from build123d import *

# Parameters (mm, degrees)
SKETCH1_W                           = 106
SKETCH1_H                           = 106
MAINOUTLINE_DEPTH                   = 1.6
SKETCH4_W                           = 11.7
SKETCH4_H                           = 11.7
RAILCUTOUTS_DEPTH                   = 2.6
FILLETCUTOUTS_START                 = -2.6
SKETCH13_W                          = 5.7
SKETCH13_H                          = 1.9
SKETCH13_W_2                        = 1.8
SKETCH13_H_2                        = 3
FILLETCUTOUTS_DEPTH                 = 3.6
SMOOTHCORNER_DEPTH                  = 10
MIRROR2_COPY_1_SKETCH_W             = 11.7
MIRROR2_COPY_1_SKETCH_H             = 11.7
MIRROR2_COPY_1_DEPTH                = 2.6
MIRROR2_START                       = -2.6
MIRROR2_COPY_2_SKETCH_W             = 5.7
MIRROR2_COPY_2_SKETCH_H             = 1.9
MIRROR2_COPY_2_SKETCH_W_2           = 1.8
MIRROR2_COPY_2_SKETCH_H_2           = 3
MIRROR2_COPY_2_DEPTH                = 3.6
MIRROR2_COPY_3_DEPTH                = 10
MIRROR2_COPY_4_SKETCH_W             = 11.7
MIRROR2_COPY_4_SKETCH_H             = 11.7
MIRROR2_COPY_4_DEPTH                = 2.6
MIRROR2_COPY_5_SKETCH_W             = 5.7
MIRROR2_COPY_5_SKETCH_H             = 1.9
MIRROR2_COPY_5_SKETCH_W_2           = 1.8
MIRROR2_COPY_5_SKETCH_H_2           = 3
MIRROR2_COPY_5_DEPTH                = 3.6
M2_CLEARANCE_HOLE1_D                = 2.1
SKETCH12_R                          = 0.8
INTERBOARDCONNECTORHOLES_DEPTH      = 1
INTERBOARDCONNECTORHOLES_DEPTH_BACK = 2.6
SKETCH16_W                          = 90
SKETCH16_H                          = 6.2
SKETCH16_W_2                        = 5.2
SKETCH16_H_2                        = 90
CUT_EXTRUDE6_DEPTH                  = 0.001
SKETCH21_R                          = 22.5
CUT_EXTRUDE10_DEPTH                 = 2.6
CUT_EXTRUDE10_DEPTH_BACK            = 1
F_2U_TURNSTILE_CUTOUT_REACH         = 3.6
SKETCH24_OUTSIDE_W                  = 137.984
SKETCH24_OUTSIDE_H                  = 137.984
SKETCH24_OUTSIDE_W_2                = 105.6
SKETCH24_OUTSIDE_H_2                = 105.6
CUT_EXTRUDE19_DEPTH                 = 2.6
FILLET7_R                           = 0.5
FILLET8_R                           = 1


with BuildPart() as part:
    # Sketch1 → mainOutline (new body)
    with BuildSketch(Plane.XY):
        Rectangle(SKETCH1_W, SKETCH1_H)
    extrude(amount=MAINOUTLINE_DEPTH)

    # Sketch4 → railCutouts (cut, through all)
    with BuildSketch(Plane(origin=(0, 0, 0), x_dir=(-1, 0, 0), z_dir=(0, 0, -1))):
        with Locations((47.15, 47.15)):
            Rectangle(SKETCH4_W, SKETCH4_H)
    railcutouts = extrude(amount=-RAILCUTOUTS_DEPTH, mode=Mode.SUBTRACT)

    # Sketch13 → filletCutouts (cut)
    with BuildSketch(Plane(origin=(0, 0, 0), x_dir=(-1, 0, 0), z_dir=(0, 0, -1)).offset(FILLETCUTOUTS_START)):
        with Locations((50.15, 40.35)):
            Rectangle(SKETCH13_W, SKETCH13_H)
        with Locations((40.4, 51.5)):
            Rectangle(SKETCH13_W_2, SKETCH13_H_2)
    filletcutouts = extrude(amount=FILLETCUTOUTS_DEPTH, mode=Mode.SUBTRACT)

    # Sketch27 → smoothCorner (cut)
    with BuildSketch(Plane.XY.offset(1.6)):
        with BuildLine():
            Line((-40.928025612, 42.198025612), (-40.928025612, 49.628025612))
            Line((-40.928025612, 49.628025612), (-40.398025612, 49.628025612))
            ThreePointArc((-40.398025612, 49.628025612), (-39.5, 50), (-39.128025612, 50.898025612))
            Line((-39.128025612, 50.898025612), (-39.128025612, 53))
            Line((-39.128025612, 53), (-53, 53))
            Line((-53, 53), (-53, 39.028025612))
            Line((-53, 39.028025612), (-48.198025612, 39.028025612))
            ThreePointArc((-48.198025612, 39.028025612), (-47.3, 39.4), (-46.928025612, 40.298025612))
            Line((-46.928025612, 40.298025612), (-46.928025612, 40.928025612))
            Line((-46.928025612, 40.928025612), (-42.198025612, 40.928025612))
            ThreePointArc((-42.198025612, 40.928025612), (-41.3, 41.3), (-40.928025612, 42.198025612))
        make_face()
    smoothcorner = extrude(amount=-SMOOTHCORNER_DEPTH, mode=Mode.SUBTRACT)

    # Mirror1: railCutouts, filletCutouts, smoothCorner across plane
    add(railcutouts.mirror(Plane(origin=(0, 0, 0), x_dir=(0, 0, 1), z_dir=(1, 0, 0))), mode=Mode.SUBTRACT)
    add(filletcutouts.mirror(Plane(origin=(0, 0, 0), x_dir=(0, 0, 1), z_dir=(1, 0, 0))), mode=Mode.SUBTRACT)
    add(smoothcorner.mirror(Plane(origin=(0, 0, 0), x_dir=(0, 0, 1), z_dir=(1, 0, 0))), mode=Mode.SUBTRACT)

    # Mirror2: smoothCorner across plane
    add(smoothcorner.mirror(Plane.ZX), mode=Mode.SUBTRACT)

    # Mirror2 copy 1 sketch → Mirror2 copy 1 (cut, through all)
    with BuildSketch(Plane(origin=(0, 0, 0), x_dir=(1, 0, 0), z_dir=(0, 0, -1))):
        with Locations((47.15, 47.15)):
            Rectangle(MIRROR2_COPY_1_SKETCH_W, MIRROR2_COPY_1_SKETCH_H)
    extrude(amount=-MIRROR2_COPY_1_DEPTH, mode=Mode.SUBTRACT)

    # Mirror2 copy 2 sketch → Mirror2 copy 2 (cut)
    with BuildSketch(Plane(origin=(0, 0, 0), x_dir=(1, 0, 0), z_dir=(0, 0, -1)).offset(MIRROR2_START)):
        with Locations((50.15, 40.35)):
            Rectangle(MIRROR2_COPY_2_SKETCH_W, MIRROR2_COPY_2_SKETCH_H)
        with Locations((40.4, 51.5)):
            Rectangle(MIRROR2_COPY_2_SKETCH_W_2, MIRROR2_COPY_2_SKETCH_H_2)
    extrude(amount=MIRROR2_COPY_2_DEPTH, mode=Mode.SUBTRACT)

    # Mirror2 copy 3 sketch → Mirror2 copy 3 (cut)
    with BuildSketch(Plane(origin=(0, 0, 1.6), x_dir=(-1, 0, 0), z_dir=(0, 0, 1))):
        with BuildLine():
            Line((-40.928025612, 42.198025612), (-40.928025612, 49.628025612))
            Line((-40.928025612, 49.628025612), (-40.398025612, 49.628025612))
            ThreePointArc((-40.398025612, 49.628025612), (-39.5, 50), (-39.128025612, 50.898025612))
            Line((-39.128025612, 50.898025612), (-39.128025612, 53))
            Line((-39.128025612, 53), (-53, 53))
            Line((-53, 53), (-53, 39.028025612))
            Line((-53, 39.028025612), (-48.198025612, 39.028025612))
            ThreePointArc((-48.198025612, 39.028025612), (-47.3, 39.4), (-46.928025612, 40.298025612))
            Line((-46.928025612, 40.298025612), (-46.928025612, 40.928025612))
            Line((-46.928025612, 40.928025612), (-42.198025612, 40.928025612))
            ThreePointArc((-42.198025612, 40.928025612), (-41.3, 41.3), (-40.928025612, 42.198025612))
        make_face()
    extrude(amount=-MIRROR2_COPY_3_DEPTH, mode=Mode.SUBTRACT)

    # Mirror2 copy 4 sketch → Mirror2 copy 4 (cut, through all)
    with BuildSketch(Plane(origin=(0, 0, 0), x_dir=(-1, 0, 0), z_dir=(0, 0, -1))):
        with Locations((47.15, -47.15)):
            Rectangle(MIRROR2_COPY_4_SKETCH_W, MIRROR2_COPY_4_SKETCH_H)
    extrude(amount=-MIRROR2_COPY_4_DEPTH, mode=Mode.SUBTRACT)

    # Mirror2 copy 5 sketch → Mirror2 copy 5 (cut)
    with BuildSketch(Plane(origin=(0, 0, 0), x_dir=(-1, 0, 0), z_dir=(0, 0, -1)).offset(MIRROR2_START)):
        with Locations((50.15, -40.35)):
            Rectangle(MIRROR2_COPY_5_SKETCH_W, MIRROR2_COPY_5_SKETCH_H)
        with Locations((40.4, -51.5)):
            Rectangle(MIRROR2_COPY_5_SKETCH_W_2, MIRROR2_COPY_5_SKETCH_H_2)
    extrude(amount=MIRROR2_COPY_5_DEPTH, mode=Mode.SUBTRACT)

    # M2 Clearance Hole1 (through all)
    with Locations(Plane(origin=(0, 0, 0), x_dir=(-1, 0, 0), z_dir=(0, 0, -1))):
        with Locations((49.5, -27.5), (27.5, -49.5), (-49.5, -27.5), (-27.5, -49.5), (-27.5, 49.5), (-49.5, 27.5), (27.5, 49.5), (49.5, 27.5)):
            Hole(M2_CLEARANCE_HOLE1_D / 2)

    # Sketch12 → interboardConnectorHoles (cut, two sides)
    with BuildSketch(Plane.XY.offset(1.6)) as interboardconnectorholes_sk:
        with Locations((27.815, -42.5)):
            Circle(SKETCH12_R)
        with Locations((38.585, -42.5)):
            Circle(SKETCH12_R)
    extrude(amount=INTERBOARDCONNECTORHOLES_DEPTH, mode=Mode.SUBTRACT)
    extrude(interboardconnectorholes_sk.sketch, amount=-INTERBOARDCONNECTORHOLES_DEPTH_BACK, mode=Mode.SUBTRACT)

    # Sketch16 → Cut-Extrude6 (cut)
    with BuildSketch(Plane.XY.offset(1.6)):
        with Locations((0, -49.9)):
            Rectangle(SKETCH16_W, SKETCH16_H)
        with Locations((0, 49.9)):
            Rectangle(SKETCH16_W, SKETCH16_H)
        with Locations((-50.4, 0)):
            Rectangle(SKETCH16_W_2, SKETCH16_H_2)
        with Locations((50.4, 0)):
            Rectangle(SKETCH16_W_2, SKETCH16_H_2)
    extrude(amount=-CUT_EXTRUDE6_DEPTH, mode=Mode.SUBTRACT)

    # Sketch21 → Cut-Extrude10 (cut, two sides)
    with BuildSketch(Plane.XY) as cut_extrude10_sk:
        Circle(SKETCH21_R)
    extrude(amount=CUT_EXTRUDE10_DEPTH, mode=Mode.SUBTRACT)
    extrude(cut_extrude10_sk.sketch, amount=-CUT_EXTRUDE10_DEPTH_BACK, mode=Mode.SUBTRACT)

    # Sketch25 → 2U turnstile cutout (cut, up to next)
    with BuildSketch(Plane(origin=(0, 0, 0), x_dir=(-1, 0, 0), z_dir=(0, 0, -1)), mode=Mode.PRIVATE) as f_2u_turnstile_cutout_sk1:
        with BuildLine():
            Line((40.937273383, -36.1866), (3.332, -36.1866))
            Line((3.332, -36.1866), (3.332, -18.4866))
            Line((3.332, -18.4866), (40.937273383, -18.4866))
            ThreePointArc((40.937273383, -18.4866), (43.19142776, -27.3366), (40.937273383, -36.1866))
        make_face()
    f_2u_turnstile_cutout_tool1 = extrude(f_2u_turnstile_cutout_sk1.sketch, amount=-F_2U_TURNSTILE_CUTOUT_REACH, mode=Mode.PRIVATE) & part.part
    add(f_2u_turnstile_cutout_tool1.solids().sort_by_distance((-22.901342, -27.3366, 0))[0], mode=Mode.SUBTRACT)
    # Sketch25 → 2U turnstile cutout (cut, up to next)
    with BuildSketch(Plane(origin=(0, 0, 0), x_dir=(-1, 0, 0), z_dir=(0, 0, -1)), mode=Mode.PRIVATE) as f_2u_turnstile_cutout_sk2:
        with BuildLine():
            Line((-18.4866, -3.332), (-18.4866, -40.937273383))
            ThreePointArc((-18.4866, -40.937273383), (-27.3366, -43.19142776), (-36.1866, -40.937273383))
            Line((-36.1866, -40.937273383), (-36.1866, -3.332))
            Line((-36.1866, -3.332), (-18.4866, -3.332))
        make_face()
    f_2u_turnstile_cutout_tool2 = extrude(f_2u_turnstile_cutout_sk2.sketch, amount=-F_2U_TURNSTILE_CUTOUT_REACH, mode=Mode.PRIVATE) & part.part
    add(f_2u_turnstile_cutout_tool2.solids().sort_by_distance((27.3366, -22.901342, 0))[0], mode=Mode.SUBTRACT)
    # Sketch25 → 2U turnstile cutout (cut, up to next)
    with BuildSketch(Plane(origin=(0, 0, 0), x_dir=(-1, 0, 0), z_dir=(0, 0, -1)), mode=Mode.PRIVATE) as f_2u_turnstile_cutout_sk3:
        with BuildLine():
            Line((-3.332, 18.4866), (-40.937273383, 18.4866))
            ThreePointArc((-40.937273383, 18.4866), (-43.19142776, 27.3366), (-40.937273383, 36.1866))
            Line((-40.937273383, 36.1866), (-3.332, 36.1866))
            Line((-3.332, 36.1866), (-3.332, 18.4866))
        make_face()
    f_2u_turnstile_cutout_tool3 = extrude(f_2u_turnstile_cutout_sk3.sketch, amount=-F_2U_TURNSTILE_CUTOUT_REACH, mode=Mode.PRIVATE) & part.part
    add(f_2u_turnstile_cutout_tool3.solids().sort_by_distance((22.901342, 27.3366, 0))[0], mode=Mode.SUBTRACT)
    # Sketch25 → 2U turnstile cutout (cut, up to next)
    with BuildSketch(Plane(origin=(0, 0, 0), x_dir=(-1, 0, 0), z_dir=(0, 0, -1)), mode=Mode.PRIVATE) as f_2u_turnstile_cutout_sk4:
        with BuildLine():
            Line((18.4866, 3.332), (18.4866, 40.937273383))
            ThreePointArc((18.4866, 40.937273383), (27.3366, 43.19142776), (36.1866, 40.937273383))
            Line((36.1866, 40.937273383), (36.1866, 3.332))
            Line((36.1866, 3.332), (18.4866, 3.332))
        make_face()
    f_2u_turnstile_cutout_tool4 = extrude(f_2u_turnstile_cutout_sk4.sketch, amount=-F_2U_TURNSTILE_CUTOUT_REACH, mode=Mode.PRIVATE) & part.part
    add(f_2u_turnstile_cutout_tool4.solids().sort_by_distance((-27.3366, 22.901342, 0))[0], mode=Mode.SUBTRACT)

    # Sketch24 outside → Cut-Extrude19 (cut, through all)
    with BuildSketch(Plane.XY.offset(1.6)):
        Rectangle(SKETCH24_OUTSIDE_W, SKETCH24_OUTSIDE_H)
        Rectangle(SKETCH24_OUTSIDE_W_2, SKETCH24_OUTSIDE_H_2, mode=Mode.SUBTRACT)
    extrude(amount=-CUT_EXTRUDE19_DEPTH, mode=Mode.SUBTRACT)

    # Fillet7
    fillet7_edges = [part.edges().sort_by_distance(p)[0] for p in [
        (-52.8, -39.028025612, 0.7995),
        (-39.128025612, -52.8, 0.7995),
        (52.8, -39.028025612, 0.7995),
        (39.128025612, 52.8, 0.7995),
        (52.8, 39.028025612, 0.7995),
        (39.128025612, -52.8, 0.7995),
        (-52.8, 39.028025612, 0.7995),
        (-39.128025612, 52.8, 0.7995),
    ]]
    fillet(fillet7_edges, radius=FILLET7_R)

    # Fillet8
    fillet8_edges = [part.edges().sort_by_distance(p)[0] for p in [
        (-36.1866, 3.332, 0.8),
        (-22.251916232, 3.332, 0.8),
        (-18.4866, 12.825584604, 0.8),
        (3.332, 36.1866, 0.8),
        (3.332, 22.251916232, 0.8),
        (12.825584604, 18.4866, 0.8),
        (36.1866, -3.332, 0.8),
        (22.251916232, -3.332, 0.8),
        (18.4866, -12.825584604, 0.8),
        (-3.332, -36.1866, 0.8),
        (-3.332, -22.251916232, 0.8),
        (-12.825584604, -18.4866, 0.8),
    ]]
    fillet(fillet8_edges, radius=FILLET8_R)


solid = part.part
Could you check a few things on this model? Use its own coordinates, in mm. A direction names the side the tool comes from. Give positions to 0.01 mm unless a question says otherwise; leave off trailing zeros. Return JSON: item names as keys, results as strings. Group by question number.
Q1. Will these pins go through, and if not, where does the flat tip stop? pin 1 Ø0.8 at (y, z) = (-45, 0.5) entering from -X; pin 2 Ø0.8 at (y, z) = (44, 1) entering from +X; pin 3 Ø0.8 at (x, z) = (-49, 1) entering from -Y.
Q2. Which directions (+Z, -Z, +X, -X, +Y, -Y) give clear straight access to the entire face, cutting with the end or side of a thin tool? Please do faces 1 (the face through (22.7, -42.6, 0.8)), 2 (the face through (-50, 1, 1.599)).
Q3. Please list where these lines run through material, in increasing order: line 1 along Y through (x, z) = (-27.5, 0.55); line 2 along Y through (x, z) = (-49.5, 0.5); line 3 along Y through (x, z) = (-18, 0.15). Write a range as [from, to].
Q4. Thinking about a two-plate mould opening in X: for faces 3 (the face through (21.03, 8, 0.79)), 4 (the face through (23, 1, 0)), which applies, pulls with the +X half, pulls with the -X half, needs draft (parallel to the pull), parting line crosses it, or undercut?
Q5. Suppose I cut it at A-A, the plane x = -31.5. State how many separate pieces and enclosed holes the cut face has, and give its area (3 significant figures).
Resolved:
{
 "1": {"pin 1": "stops at x = -40.93", "pin 2": "stops at x = 40.93", "pin 3": "stops at y = -39.03"},
 "2": {"face 1": "+Z, -Z", "face 2": "+Z, +X, -X, +Y, -Y"},
 "3": {"line 1": "y = [-52.8, -50.55], [-48.45, -36.19], [-18.49, 3.33], [43.19, 48.45], [50.55, 52.8]", "line 2": "y = [-39.03, -28.55], [-26.45, 26.45], [28.55, 39.03]", "line 3": "y = [-52.8, -36.19], [-18.49, -13.5], [14.84, 52.8]"},
 "4": {"face 3": "undercut", "face 4": "needs draft"},
 "5": {"separate pieces": "3", "enclosed holes": "0", "area": "77.6 mm2"}
}
